```python
from build123d import *

# Parameters (mm, degrees)
BOSS_EXTRUDE1_DEPTH = 5
CHAMFER1_SIZE       = 0.2


with BuildPart() as part:
    # Sketch1 → Boss-Extrude1 (new body)
    with BuildSketch(Plane(origin=(0, 0, 0), x_dir=(1, 0, 0), z_dir=(0, 1, 0))):
        with BuildLine():
            Line((-5, 30.807690886), (5, 30.807690886))
            Line((5, 30.807690886), (5, 20.807690886))
            ThreePointArc((5, 20.807690886), (19.662998381, 8.445501445), (18.532943641, -10.7))
            ThreePointArc((18.532943641, -10.7), (15.117880132, -11.615063509), (14.202816622, -8.2))
            ThreePointArc((14.202816622, -8.2), (0, 16.4), (-14.202816622, -8.2))
            ThreePointArc((-14.202816622, -8.2), (-15.117880132, -11.615063509), (-18.532943641, -10.7))
            ThreePointArc((-18.532943641, -10.7), (-19.662998381, 8.445501445), (-5, 20.807690886))
            Line((-5, 20.807690886), (-5, 30.807690886))
        make_face()
    extrude(amount=BOSS_EXTRUDE1_DEPTH)

    # Chamfer1
    chamfer1_edges = [part.edges().sort_by_distance(p)[0] for p in [
        (15.117880132, 0, 11.615063509),
        (0, 0, -16.4),
        (-15.117880132, 0, 11.615063509),
        (-19.662998381, 0, -8.445501445),
        (0, 5, -16.4),
        (15.117880132, 5, 11.615063509),
        (19.662998381, 5, -8.445501445),
        (5, 5, -25.807690886),
        (0, 5, -30.807690886),
        (-5, 5, -25.807690886),
        (-19.662998381, 5, -8.445501445),
        (-5, 0, -25.807690886),
        (-15.117880132, 5, 11.615063509),
        (0, 0, -30.807690886),
        (5, 0, -25.807690886),
        (19.662998381, 0, -8.445501445),
    ]]
    chamfer(chamfer1_edges, length=CHAMFER1_SIZE)


solid = part.part
```
The listing builds one solid part. Answer for the finished solid, in the listing's coordinates (mm). A direction names the side the tool comes from. Give positions to 0.01 mm unless a question says otherwise; leave off trailing zeros. Order: outer loops, then holes, each group sorted by start corner. A loop starts at its lowest first (then second) coordinate and runs counter-clockwise, first axis right, second up. Notation, with made-up numbers: (45, -30.75) -> (68, -30.75) arc R22 cw to (68, -23.75) -> close; hole circle Ø8 at (9.25, 5). An arc over 180 degrees is marked (long way). Write each question's results on one line, items separated by ' | '.
Q1. The part is cut by section B-B, the plane x = 0. Give the vertices of the cut face in (y, z).
Checked values:
outline: (0, -30.61) -> (0.2, -30.81) -> (4.8, -30.81) -> (5, -30.61) -> (5, -16.6) -> (4.8, -16.4) -> (0.2, -16.4) -> (0, -16.6) -> close
Q2. This flat-tipped pin is pushed along its axis until it touches: P1, Ø1, axis at x = -8, y = 2.5, coming from the -Z side. Where does it stop, or does it pass through?
Checked values:
P1: stops at z = -20.04
Q3. Straight lines are drawn through the part: probe 1 along X at (y, z) = (1.8, 0); probe 2 along Z at (x, y) = (0, 2.05); probe 3 along X at (y, z) = (0.2, -24). For each, find the intervals that lie inside material, in ascending order. Write a range as from..to.
Checked values:
probe 1: x = -21.4..-16.4, 16.4..21.4 | probe 2: z = -30.81..-16.4 | probe 3: x = -5..5
Q4. The part is cut by section A-A, the plane z = 0. Give the vertices of the cut face in (x, y).
Checked values:
outline: (-21.4, 0.2) -> (-21.2, 0) -> (-16.6, 0) -> (-16.4, 0.2) -> (-16.4, 4.8) -> (-16.6, 5) -> (-21.2, 5) -> (-21.4, 4.8) -> close; (16.4, 0.2) -> (16.6, 0) -> (21.2, 0) -> (21.4, 0.2) -> (21.4, 4.8) -> (21.2, 5) -> (16.6, 5) -> (16.4, 4.8) -> close
Q5. The part is cut by section C-C, the plane z = -23. Give the vertices of the cut face in (x, y), and give its area (3 significant figures).
Checked values:
outline: (-5, 0.2) -> (-4.8, 0) -> (4.8, 0) -> (5, 0.2) -> (5, 4.8) -> (4.8, 5) -> (-4.8, 5) -> (-5, 4.8) -> close | area: 49.9 mm^2
Q6. Determine the mould class of faces 1 (the face through (0, 2, -30.808)), 2 (the face through (-15.071, 2.468, 11.587)), 3 (the face through (-5, 2, -26)) for opening direction Z: pulls with the +Z half, pulls with the -Z half, needs draft (parallel to the pull), parting line crosses it, or undercut.
Checked values:
face 1: pulls with the -Z half | face 2: undercut | face 3: needs draft
Q7. Which of the six approach directions +Z, -Z, +X, -X, +Y, -Y give full straight-line access (tool end or side, diameter ignored) to faces 4 (the face through (5, 2, -26)), 5 (the face through (-19.77, 2.47, -8.19))?
Checked values:
face 4: -Z, +X, +Y, -Y | face 5: -X, +Y, -Y
